Input: part model. Units: mm. Frame: model coordinates. Coordinates: 2 decimals unless noted, no trailing zeros. Loops run counter-clockwise (first coordinate to the right, second up) from the corner with the lowest first, then second, coordinate; pieces in that order, holes last.
(1) Mould query, pull axis Y, two halves, no side actions, for faces 1 (the face through (0, 5, -7)), 2 (the face through (-1.19, -5.37, -3.45)), 3 (the face through (-0.867, -3.905, -3.459)). Classes: released by +Y, released by -Y, zero draft, split by the parting line, or undercut.
(2) Section C-C, the plane z = -5. Return loops of the section in (x, y), then the cut area to 3 significant figures.
(3) Line query: L1, parallel to Y at x = 0, z = -2.8; L2, parallel to Y at x = 3, z = -2.5; L3, parallel to X at y = -1.25, z = -5.25. Output: solid intervals per line, ascending.
(4) Section A-A, the plane x = 0. Return loops of the section in (y, z).
Autodesk Inventor part; units mm, degrees
ref_plane "YZ Plane" through (0, 0, 0) normal (1, 0, 0) x (0, 1, 0)
ref_plane "XZ Plane" through (0, 0, 0) normal (0, 1, 0) x (-1, 0, 0)
ref_plane "XY Plane" through (0, 0, 0) normal (0, 0, 1) x (1, 0, 0)
sketch "Sketch1" plane through (0, 0, 0) normal (0, 0, 1) x (1, 0, 0)
  circle A0 centre (0, 0) radius 5.5
  circle A1 centre (0, 0) radius 4
  dimension "d0" = 11
  dimension "d1" = 8
extrude "Extrusion1" add sketch "Sketch1" against normal blind 7
chamfer "Chamfer1" distance 0.6 angle 45 2 edges at (-4, 0, 0) (-4, 0, -7)
chamfer "Chamfer2" distance 0.2 angle 45 2 edges at (-5.5, 0, -7) (-5.5, 0, 0)
properties part number "608-inner"
Report:
1. face 1: zero draft
1. face 2: split by the parting line
1. face 3: undercut
2. outline: circle Ø11 at (0, 0); hole circle Ø8 at (0, 0)
2. area: 44.8 mm2
3. L1: y = -5.5 to -4, 4 to 5.5
3. L2: y = -4.61 to -2.65, 2.65 to 4.61
3. L3: x = -5.36 to -3.8, 3.8 to 5.36
4. outline: (-5.5, -6.8) - (-5.3, -7) - (-4.6, -7) - (-4, -6.4) - (-4, -0.6) - (-4.6, 0) - (-5.3, 0) - (-5.5, -0.2) - close; (4, -6.4) - (4.6, -7) - (5.3, -7) - (5.5, -6.8) - (5.5, -0.2) - (5.3, 0) - (4.6, 0) - (4, -0.6) - close
